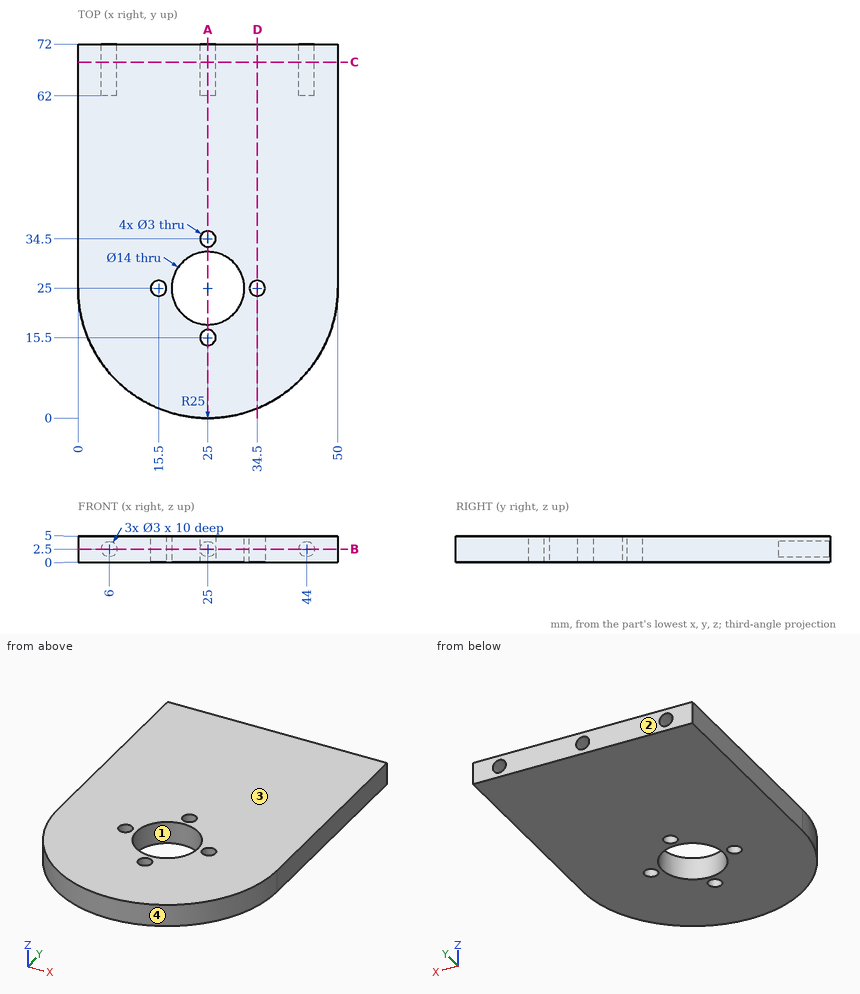
The figure shows three views and two pictorial views of one solid part (mm, origin at its lowest corner). Answer the questions. Coordinates: 2 decimals unless noted, no trailing zeros. Loops run counter-clockwise (first coordinate to the right, second up) from the corner with the lowest first, then second, coordinate; pieces in that order, holes last. Notation, with made-up numbers: (-29.75, 56.5) -> (-19.75, 56.5) arc R12 ccw to (-19.75, 71.5) -> close; hole circle Ø7 at (86, -30). An arc over 180 degrees is marked (long way). Write item = value, one per line. Start each with the question number.
1) Given pin 1 Ø1 at (x, z) = (28.5, 0.5) entering from -Y; pin 2 Ø1.8 at (x, z) = (6, 2.5) entering from +Y; pin 3 Ø18 at (x, y) = (25, 25) entering from +Z; pin 4 Ø2 at (y, z) = (22, 3.5) entering from +X, each flat-ended and moving along its own axis, determine where each tip first touches the part or whether it passes through.
2) A cutting plane is placed at C-C (y = 68.5). Give the vertices of the cut face in (x, z), then the cut area to 3 significant figures.
3) A cutting plane is placed at D-D (x = 34.5). Give the vertices of the cut face in (y, z).
4) The mould has two halves that part along Y. Classify the marked faces 1, 2, 3 and 4: released by +Y, released by -Y, zero draft, split by the parting line, or undercut.
5) A cutting plane is placed at B-B (z = 2.5). Give the vertices of the cut face in (x, y), then the cut area to 3 significant figures.
6) A cutting plane is placed at A-A (x = 25). Give the vertices of the cut face in (y, z), then the cut area to 3 significant figures.
7) Straight lines are drawn through the part: line 1 (X direction, y = 69.5, z = 2.5); line 2 (Y direction, x = 25, z = 1.15); line 3 (X direction, y = 31, z = 4.45). For each, find the intervals that lie inside material, in ascending order. Write a range as from..to.
Responses:
q1.pin_1 = 0.18
q1.pin_2 = 62
q1.pin_3 = 5
q1.pin_4 = 49.92
q2.outline = (0, 0) -> (50, 0) -> (50, 5) -> (0, 5) -> close; hole circle Ø3 at (6, 2.5); hole circle Ø3 at (25, 2.5); hole circle Ø3 at (44, 2.5)
q2.area = 229 mm²
q3.outline = (1.88, 0) -> (23.5, 0) -> (23.5, 5) -> (1.88, 5) -> close; (26.5, 0) -> (72, 0) -> (72, 5) -> (26.5, 5) -> close
q4.face_1 = undercut
q4.face_2 = released by +Y
q4.face_3 = zero draft
q4.face_4 = released by -Y
q5.outline = (0, 25) arc R25 ccw to (50, 25) -> (50, 72) -> (45.5, 72) -> (45.5, 62) -> (42.5, 62) -> (42.5, 72) -> (26.5, 72) -> (26.5, 62) -> (23.5, 62) -> (23.5, 72) -> (7.5, 72) -> (7.5, 62) -> (4.5, 62) -> (4.5, 72) -> (0, 72) -> close; hole circle Ø3 at (15.5, 25); hole circle Ø14 at (25, 25); hole circle Ø3 at (25, 15.5); hole circle Ø3 at (25, 34.5); hole circle Ø3 at (34.5, 25)
q5.area = 3,060 mm²
q6.outline = (0, 0) -> (14, 0) -> (14, 5) -> (0, 5) -> close; (17, 0) -> (18, 0) -> (18, 5) -> (17, 5) -> close; (32, 0) -> (33, 0) -> (33, 5) -> (32, 5) -> close; (36, 0) -> (72, 0) -> (72, 1) -> (62, 1) -> (62, 4) -> (72, 4) -> (72, 5) -> (36, 5) -> close
q6.area = 230 mm²
q7.line_1 = 0..4.5, 7.5..23.5, 26.5..42.5, 45.5..50
q7.line_2 = 0..14, 17..18, 32..33, 36..62
q7.line_3 = 0..21.39, 28.61..50
